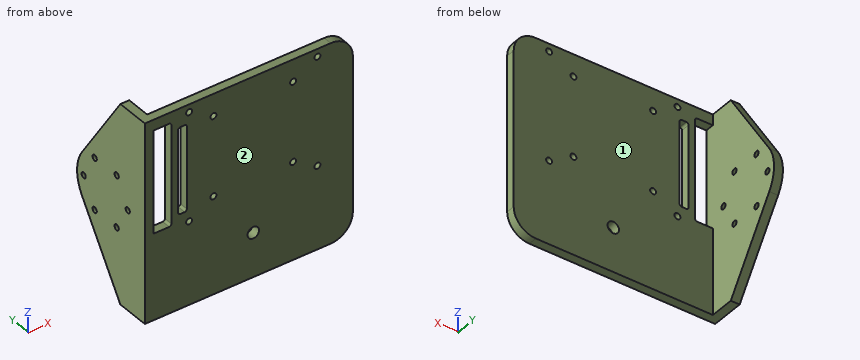
```python
from build123d import *

# Parameters (mm, degrees)
SKETCH_3_W          = 90
SKETCH_3_H          = 90
EXTRUDE_3_DEPTH     = 4
EXTRUDE_4_DEPTH     = 4
SKETCH_5_R          = 1.3
CUT_EXTRUDE_1_DEPTH = 4
SKETCH_6_R          = 2.6
SKETCH_6_R_2        = 1.35
CUT_EXTRUDE_2_DEPTH = 4
SKETCH_7_W          = 4
SKETCH_7_H          = 39
SKETCH_7_W_2        = 8
SKETCH_7_H_2        = 46.3
CUT_EXTRUDE_3_DEPTH = 4
FILLET_3_R          = 1
FILLET_4_R          = 10


with BuildPart() as part:
    # 草图3 → 凸台-拉伸3 (new body)
    with BuildSketch(Plane(origin=(0, 0, 0), x_dir=(1, 0, 0), z_dir=(0, 1, 0))):
        Rectangle(SKETCH_3_W, SKETCH_3_H)
    extrude(amount=EXTRUDE_3_DEPTH)

    # 草图4 → 凸台-拉伸4 (add)
    with BuildSketch(Plane.ZY.offset(45)):
        with BuildLine():
            Line((-45, 4), (-45, 15))
            Line((-45, 15), (-9.716498114, 38.55471279))
            ThreePointArc((-9.716498114, 38.55471279), (0, 41.5), (9.716498114, 38.55471279))
            Line((9.716498114, 38.55471279), (45, 15))
            Line((45, 15), (45, 4))
            Line((45, 4), (45, 0))
            Line((45, 0), (-45, 0))
            Line((-45, 0), (-45, 4))
        make_face()
    extrude(amount=EXTRUDE_4_DEPTH)

    # 草图5 → 切除-拉伸1 (cut)
    with BuildSketch(Plane(origin=(-45, 0, 0), x_dir=(0, 0, -1), z_dir=(1, 0, 0))):
        with Locations((0, 37.5)):
            Circle(SKETCH_5_R)
        with Locations((11.691342951, 30.75)):
            Circle(SKETCH_5_R)
        with Locations((11.691342951, 17.25)):
            Circle(SKETCH_5_R)
        with Locations((0, 10.5)):
            Circle(SKETCH_5_R)
        with Locations((-11.691342951, 17.25)):
            Circle(SKETCH_5_R)
        with Locations((-11.691342951, 30.75)):
            Circle(SKETCH_5_R)
    extrude(amount=-CUT_EXTRUDE_1_DEPTH, mode=Mode.SUBTRACT)

    # 草图6 → 切除-拉伸2 (cut)
    with BuildSketch(Plane(origin=(0, 4, 0), x_dir=(1, 0, 0), z_dir=(0, 1, 0))):
        with Locations(Location((0, 25.05, 0), (0, 0, 270))):
            Circle(SKETCH_6_R)
        with Locations(Location((-29, -41.5, 0), (0, 0, 270))):
            Circle(SKETCH_6_R_2)
        with Locations(Location((-29, 7.5, 0), (0, 0, 270))):
            Circle(SKETCH_6_R_2)
        with Locations(Location((-18, -35, 0), (0, 0, 270))):
            Circle(SKETCH_6_R_2)
        with Locations(Location((-18, 1, 0), (0, 0, 270))):
            Circle(SKETCH_6_R_2)
        with Locations(Location((29, -41.5, 0), (0, 0, 90))):
            Circle(SKETCH_6_R_2)
        with Locations(Location((18, -35, 0), (0, 0, 90))):
            Circle(SKETCH_6_R_2)
        with Locations(Location((18, 1, 0), (0, 0, 90))):
            Circle(SKETCH_6_R_2)
        with Locations(Location((29, 7.5, 0), (0, 0, 90))):
            Circle(SKETCH_6_R_2)
    extrude(amount=-CUT_EXTRUDE_2_DEPTH, mode=Mode.SUBTRACT)

    # 草图7 → 切除-拉伸3 (cut)
    with BuildSketch(Plane(origin=(0, 4, 0), x_dir=(1, 0, 0), z_dir=(0, 1, 0))):
        with Locations((-32, -17)):
            Rectangle(SKETCH_7_W, SKETCH_7_H)
        with Locations((-41, -17)):
            Rectangle(SKETCH_7_W_2, SKETCH_7_H_2)
    extrude(amount=-CUT_EXTRUDE_3_DEPTH, mode=Mode.SUBTRACT)

    # 圆角3
    fillet_3_edges = [part.edges().sort_by_distance(p)[0] for p in [
        (-37, 2, 40.15),
        (-37, 2, -6.15),
        (-30, 2, 36.5),
        (-30, 2, -2.5),
        (-34, 2, -2.5),
        (-34, 2, 36.5),
    ]]
    fillet(fillet_3_edges, radius=FILLET_3_R)

    # 圆角4
    fillet_4_edges = [part.edges().sort_by_distance(p)[0] for p in [
        (45, 2, 45),
        (45, 2, -45),
    ]]
    fillet(fillet_4_edges, radius=FILLET_4_R)


solid = part.part
```
Geometry: final body of the model. Coordinates: model frame, mm. Face numbers are marked on the shaded views. A direction names the side the tool comes from. Coordinates: 2 decimals unless noted, no trailing zeros. Order: outer loops, then holes, each group sorted by start corner. A loop starts at its lowest first (then second) coordinate and runs counter-clockwise, first axis right, second up.
Item 1: Material intervals for line 1 along X through (y, z) = (3, -1); line 2 along Y through (x, z) = (-46.35, 0); line 3 along X through (y, z) = (1.6, -7.5), sorted ascending.
Answer:
line 1: x = -49 to -45, -37 to -34, -30 to -19.35, -16.65 to 16.65, 19.35 to 45
line 2: y = 0 to 9.2, 11.8 to 36.2, 38.8 to 41.5
line 3: x = -49 to -30.35, -27.65 to 27.65, 30.35 to 45
Item 2: Section query A-A (x = 18). Output: boundary loops of the cut face in (y, z).
Answer:
outline: (0, -45) - (4, -45) - (4, -2.35) - (0, -2.35) - close; (0, 0.35) - (4, 0.35) - (4, 33.65) - (0, 33.65) - close; (0, 36.35) - (4, 36.35) - (4, 45) - (0, 45) - close
Item 3: Section query D-D (y = 7). Output: boundary loops of the cut face in (x, z), then the cut area to 3 significant figures.
Answer:
outline: (-49, -45) - (-45, -45) - (-45, 45) - (-49, 45) - close
area: 360 mm2
Item 4: Section query B-B (z = 24). Output: boundary loops of the cut face in (x, y), then the cut area to 3 significant figures.
Answer:
outline: (-49, 0) - (-45, 0) - (-45, 29.02) - (-49, 29.02) - close; (-37, 0) - (-34, 0) - (-34, 4) - (-37, 4) - close; (-30, 0) - (45, 0) - (45, 4) - (-30, 4) - close
area: 428 mm2
Item 5: Section query C-C (z = -25.05). Output: boundary loops of the cut face in (x, y).
Answer:
outline: (-49, 0) - (-2.6, 0) - (-2.6, 4) - (-45, 4) - (-45, 28.32) - (-49, 28.32) - close; (2.6, 0) - (45, 0) - (45, 4) - (2.6, 4) - close
Item 6: Access query for the marked faces 1 and 2. Directions: +Z, -Z, +X, -X, +Y, -Y. A direction counts if a zero-diameter tool reaches every point of the face in a straight line with its end or side. Return the directions, or none.
Answer:
face 1: +Z, -Z, +X, +Y
face 2: +Z, -Z, +X, -X, -Y
Item 7: Contact query for flat-ended pins moving along their axis: P1, Ø2, axis at x = 18, z = 35, coming from the -Y side; P2, Ø12, axis at x = -28, z = 13, coming from the +Y side; P3, Ø10, axis at y = 29.5, z = 26.5, coming from the +X side. Output: stop coordinate, or through.
Answer:
P1: passes through
P2: stops at y = 4
P3: stops at x = -45
